Check sheet for the modelled part. Datum: model origin and axes. Units: mm. A direction names the side the tool comes from. Coordinates: 2 decimals unless noted, no trailing zeros. Loops run counter-clockwise (first coordinate to the right, second up) from the corner with the lowest first, then second, coordinate; pieces in that order, holes last. Notation, with made-up numbers: M 34.5,-31.5 L 51.5,-31.5 A19 cw 51.5,0.5 Z; hole C 17.25,48 d2. An arc over 180 degrees is marked long. Return JSON: item names as keys, results as strings.
Autodesk Inventor part; units mm, degrees
ref_plane "YZ Plane" through (0, 0, 0) normal (1, 0, 0) x (0, 1, 0)
ref_plane "XZ Plane" through (0, 0, 0) normal (0, 1, 0) x (-1, 0, 0)
ref_plane "XY Plane" through (0, 0, 0) normal (0, 0, 1) x (1, 0, 0)
sketch "Sketch1" plane through (0, 0, 0) normal (0, 1, 0) x (-1, 0, 0)
  line L0 (0, 0) -> (0, -40)
  line L1 (0, -40) -> (4, -40)
  line L2 (4, -40) -> (4, -8.4853)
  line L3 (4, -8.4853) -> (9.6569, -14.1421)
  line L4 (9.6569, -14.1421) -> (13.8995, -9.8995)
  line L5 (13.8995, -9.8995) -> (4, 0)
  line L6 (4, 0) -> (0, 0)
  dimension "d0" = 45
  dimension "d1" = 4
  dimension "d2" = 40
  dimension "d12" = 6
  dimension "d13" = 8
  dimension "d14" = 4
extrude "Extrusion1" add sketch "Sketch1" along normal blind 6
sketch "Sketch2" plane through (-13.8995, 0, -9.8995) normal (-0.7071, 0, -0.7071) x (-0.7071, 0, 0.7071)
  line L0 (-2.8284, 0) -> (-2.8284, 6)
  line L1 (-6, 0) -> (0, 0)
  line L2 (0, 0) -> (0, 6)
  line L3 (-6, 6) -> (0, 6)
  line L4 (-6, 0) -> (-6, 6)
  circle A0 centre (-3.416, 3) radius 0.65
  dimension "d5" = 1.3
  dimension "d6" = 3
extrude "Extrusion2" cut sketch "Sketch2" against normal blind 15 contours A0 L0 | L0 A0
fillet "Fillet1" radius 2 1 edges at (-4, 3, -8.4853)
fillet "Fillet2" radius 2 6 edges at (-8.5355, 6, -13.0208) (-4, 6, -26.6569) (-8.5355, 0, -13.0208) (-4, 0, -26.6569) (-8.9497, 6, -4.9497) (-8.9497, 0, -4.9497)
properties part number "AntennaAdapter" material "ABS Plastic"
1) Section check C-C on y = 0.95. Record the cut outline in (x, z), then the cut area to 3 significant figures.
Answers:
{"outline": "M -13.69,-10.11 L -9.87,-13.93 L -7.62,-11.69 A2.3 cw -3.7,-13.31 L -3.7,-40 L 0,-40 L 0,0 L -3.58,0 Z", "area": "216 mm²"}
2) Set-up check for faces 1 (the face through (-8.52, 2.986, -13.005)), 2 (the face through (-8.95, 0.6, -12.63)), 3 (the face through (-8.977, 5.43, -12.611)), 4 (the face through (-0.87, 3.009, -1.713)): record each of +Z, -Z, +X, -X, +Y, -Y from which the full face is reachable in a straight line by a thin tool's end or side.
Answers:
{"face 1": "-Z, +Y, -Y", "face 2": "-Z, -Y", "face 3": "-Z, +Y", "face 4": "none"}
3) Section check B-B on y = 5.25. Record the cut outline in (x, z), then the cut area to 3 significant figures.
Answers:
{"outline": "M -13.59,-10.21 L -9.97,-13.83 L -7.72,-11.59 A2.44 cw -3.56,-13.31 L -3.56,-40 L 0,-40 L 0,0 L -3.38,0 Z", "area": "209 mm²"}
4) Scan lines: line 1 along X through (y, z) = (2.7, -23.5); line 2 along Z through (x, y) = (-7, 3.1); line 3 along Z through (x, y) = (-2, 3.1). Record each from-to range of solid material in increasing order. Write a range as [from, to].
Answers:
{"line 1": "[-4, 0]", "line 2": "[-11.58, -8.74], [-6.92, -3]", "line 3": "[-40, -3.74], [-1.92, 0]"}
5) Draft check along Z on faces 5 (the face through (-9, 3, -5)), 6 (the face through (-1.6, 0, -15.5)), 7 (the face through (-6.155, 2.365, -7.185)). Enter one of: +Z half, -Z half, draft (parallel to the pull), parting line (faces both ways), or undercut.
Answers:
{"face 5": "+Z half", "face 6": "draft", "face 7": "undercut"}
6) Section check A-A on z = -33. Record the cut outline in (x, y), then the cut area to 3 significant figures.
Answers:
{"outline": "M -4,2 A2 ccw -2,0 L 0,0 L 0,6 L -2,6 A2 ccw -4,4 Z", "area": "22.3 mm²"}
7) Go/stop test with flat-tipped pins: pin 1 Ø1.5 at (y, z) = (1.5, -4.5) entering from +X; pin 2 Ø1.6 at (y, z) = (3.5, -24) entering from -X; pin 3 Ø1 at (x, y) = (-12.5, 4) entering from -Z; pin 4 Ø3 at (x, z) = (-7, -21) entering from +Y. Record where each tip stops, or that it passes through.
Answers:
{"pin 1": "x = 0", "pin 2": "x = -4", "pin 3": "z = -11.8", "pin 4": "through"}
